Geometry check sheet. Reference: the model listing, model coordinates, mm. Coordinates: 2 decimals unless noted, no trailing zeros. Write each loop counter-clockwise with the first axis right and the second up, starting at its lowest first coordinate (ties: lowest second). Pieces come first, ordered by that corner, then holes. Notation, with made-up numbers: (-10, 14) -> (0, 14) arc R9 cw to (0, 29) -> close; hole circle Ø5 at (35.5, -28.75). An arc over 180 degrees is marked (long way). Answer in a Markdown table with one row per item. Add a question column.
Q1. Section check A-A, the plane x = -210. Record the boundary of the cut face in (y, z), and give its area (4 significant figures).
Q2. Thickness scan on line 1 (X direction, y = -191, z = -4.25); line 2 (Y direction, x = -35, z = -4.75); line 3 (Z direction, x = -436.5, y = -576). Record the ranges inside material, lowest first.
Q3. Section check B-B, the plane y = -170.5. Record the boundary of the cut face in (x, z).
Q4. Gauge pin test, flat ends, axial feed: P1, Ø1.5, axis at x = -352.5, z = -3, coming from the +Y side; P2, Ø8, axis at x = -432, y = -295.5, coming from the +Z side. Record the tip position at first contact, or that the pin passes through.
Q5. Release check for a two-part mould opening along Y. For faces 1 (the face through (-304, 0, -9)), 2 (the face through (-303, -371, -5)), 3 (the face through (-304, -750, -9)), 4 (the face through (-304, -370, -18)) record: pulls with the +Y half, pulls with the -Y half, needs draft (parallel to the pull), parting line crosses it, or undercut.
```python
from build123d import *

# Parameters (mm, degrees)
SCHIZZO1_W         = 600
SCHIZZO1_H         = 750
PANNELLO_DEPTH     = 18
SCHIZZO2_R         = 2.5
FOROMANIGLIA_DEPTH = 961.637288471
SCHIZZO3_W         = 460
SCHIZZO3_H         = 610
LAVORAZIONE_DEPTH  = 5


with BuildPart() as part:
    # Schizzo1 → Pannello (new body)
    with BuildSketch(Plane.XY):
        with Locations((-300, -375)):
            Rectangle(SCHIZZO1_W, SCHIZZO1_H)
    extrude(amount=-PANNELLO_DEPTH)

    # Schizzo2 → ForoManiglia (cut, through all)
    with BuildSketch(Plane.XY):
        with Locations((-35, -70)):
            Circle(SCHIZZO2_R)
    extrude(amount=-FOROMANIGLIA_DEPTH, mode=Mode.SUBTRACT)

    # Schizzo3 → Lavorazione (cut)
    with BuildSketch(Plane.XY):
        with Locations((-300, -375)):
            Rectangle(SCHIZZO3_W, SCHIZZO3_H)
    extrude(amount=-LAVORAZIONE_DEPTH, mode=Mode.SUBTRACT)


solid = part.part
```
Calculated:
| question | item | result |
|---|---|---|
| 1 | outline | (-750, -18) -> (0, -18) -> (0, 0) -> (-70, 0) -> (-70, -5) -> (-680, -5) -> (-680, 0) -> (-750, 0) -> close |
| 1 | area | 10,450 mm² |
| 2 | line 1 | x = -600 to -530, -70 to 0 |
| 2 | line 2 | y = -750 to -72.5, -67.5 to 0 |
| 2 | line 3 | z = -18 to -5 |
| 3 | outline | (-600, -18) -> (0, -18) -> (0, 0) -> (-70, 0) -> (-70, -5) -> (-530, -5) -> (-530, 0) -> (-600, 0) -> close |
| 4 | P1 | stops at y = 0 |
| 4 | P2 | stops at z = -5 |
| 5 | face 1 | pulls with the +Y half |
| 5 | face 2 | undercut |
| 5 | face 3 | pulls with the -Y half |
| 5 | face 4 | needs draft |
